from build123d import *

# Parameters (mm, degrees)
SKETCH1_R           = 3.06
BOSS_EXTRUDE1_DEPTH = 2
BOSS_EXTRUDE3_DEPTH = 5
SKETCH6_W           = 56
SKETCH6_H           = 2
BOSS_EXTRUDE4_DEPTH = 2
FILLET2_R           = 30
FILLET3_R           = 4


with BuildPart() as part:
    # Sketch1 → Boss-Extrude1 (new body)
    with BuildSketch(Plane(origin=(0, 0, 0), x_dir=(1, 0, 0), z_dir=(0, 1, 0))):
        with BuildLine():
            Line((-5, 0), (-5, 5))
            Line((-5, 5), (71, 5))
            Line((71, 5), (71, -3))
            ThreePointArc((71, -3), (66, -8), (61, -3))
            Line((61, -3), (61, 3.06))
            Line((61, 3.06), (5, 3.06))
            Line((5, 3.06), (5, 0))
            ThreePointArc((5, 0), (0, -5), (-5, 0))
        make_face()
        with Locations(Location((0, 0, 0), (0, 0, 270))):
            Circle(SKETCH1_R, mode=Mode.SUBTRACT)
        with Locations(Location((66, -3, 0), (0, 0, 270))):
            Circle(SKETCH1_R, mode=Mode.SUBTRACT)
    extrude(amount=BOSS_EXTRUDE1_DEPTH)

    # Sketch4 → Boss-Extrude3 (add)
    with BuildSketch(Plane(origin=(0, 0, 0), x_dir=(-1, 0, 0), z_dir=(0, -1, 0))):
        Polygon((5, 5), (-71, 5), (-89.933264969, -12.968832246), (-66.5, 3.06), (5, 3.06), align=None)
    extrude(amount=BOSS_EXTRUDE3_DEPTH)

    # Sketch6 → Boss-Extrude4 (add)
    with BuildSketch(Plane(origin=(0, 2, 0), x_dir=(1, 0, 0), z_dir=(0, 1, 0))):
        with Locations((33, 2.06)):
            Rectangle(SKETCH6_W, SKETCH6_H)
    extrude(amount=-BOSS_EXTRUDE4_DEPTH)

    # Fillet2
    # the kernel refuses this fillet: 30 mm, written as the material it takes off along each edge
    with BuildSketch(Plane(origin=(71, 29.924182181, -5), x_dir=(0.7253392750671382, 0, 0.6883915572151349), z_dir=(0, -1, 0))) as fillet2_piece_1:
        with BuildLine():
            CenterArc((FILLET2_R * 0.398989095747, FILLET2_R), FILLET2_R, 226.497078838, 43.502921162)
            Line((-FILLET2_R * 0.289402461469, FILLET2_R * 0.274660724933), (0, 0))
            Line((0, 0), (FILLET2_R * 0.398989095747, 0))
        make_face()
    extrude(amount=64.848364362, mode=Mode.SUBTRACT)

    # Fillet3
    # the kernel refuses this fillet: 4 mm, written as the material it takes off along each edge
    with BuildSketch(Plane(origin=(-5, 12, -5), x_dir=(0, 0, 1), z_dir=(0, -1, 0))) as fillet3_piece_1:
        with BuildLine():
            CenterArc((FILLET3_R, -FILLET3_R), FILLET3_R, 90, 90)
            Line((0, -FILLET3_R), (0, 0))
            Line((0, 0), (FILLET3_R, 0))
        make_face()
    extrude(amount=27, mode=Mode.SUBTRACT)


solid = part.part
Verification items for the finished model (mm, model axes). A direction names the side the tool comes from. Round coordinates to 2 decimals unless told otherwise and drop trailing zeros. Loops run counter-clockwise (first coordinate to the right, second up) from the corner with the lowest first, then second, coordinate; pieces in that order, holes last. Notation, with made-up numbers: M -31,-9.75 L -7,-9.75 A20 cw -7,9.25 Z; hole C -36,-35.75 d1. An arc over 180 degrees is marked long. Write each question's results on one line, items separated by ' | '.
1) Scan lines: L1, parallel to Z at x = 15, y = -2.75; L2, parallel to Y at x = 63, z = -3; L3, parallel to X at y = 1, z = 3.25. Record each from-to range of solid material in increasing order. Write a range as from..to.
Checks:
L1: z = -5..-3.06 | L2: y = 0..2 | L3: x = -3.8..3.8, 61.01..62.95, 69.05..70.99
2) Access from +Z, -Z, +X, -X, +Y, -Y to the whole of each face (thin tool, end or side, straight path). Record for faces 1 (the flat face through (36, 0, -2)), 2 (the cylindrical face through (-2.99, 0.99, -0.66)), 3 (the flat face through (78, 0, 3)), 4 (the flat face through (33, 1, -1.06)).
Checks:
face 1: +Z, -X, -Y | face 2: +Y, -Y | face 3: +Z, -Z, +X, +Y | face 4: +Z, +Y, -Y
3) Section check A-A on z = 7. Record the boundary of the cut face in (x, y), then the cut area to 3 significant figures.
Checks:
outline: M 63,0 L 69,0 L 69,2 L 63,2 Z; M 81.21,-5 L 83.64,-5 L 83.64,0 L 81.21,0 Z | area: 24.2 mm2
4) Section check D-D on x = 80.5. Record the boundary of the cut face in (y, z).
Checks:
outline: M -5,4.02 L 0,4.02 L 0,6.52 L -5,6.52 Z
5) Mould release check, pull along Z, two halves, no side actions. Record for faces 5 (the cylindrical face through (63.01, 0.99, 2.34)), 6 (the flat face through (71, 1, 0)), 7 (the flat face through (78.381, -2.465, 5.067)): released by +Z, released by -Z, zero draft, split by the parting line, or undercut.
Checks:
face 5: undercut | face 6: zero draft | face 7: released by +Z
6) Section check C-C on y = -1. Record the boundary of the cut face in (x, z).
Checks:
outline: M -4.43,-3.06 A4 ccw -1,-5 L 59.03,-5 A30 ccw 79.68,3.24 L 89.93,12.97 L 66.5,-3.06 Z
7) Section check B-B on x = 26. Record the boundary of the cut face in (y, z), then the cut area to 3 significant figures.
Checks:
outline: M -5,-5 L 2,-5 L 2,-1.06 L 0,-1.06 L 0,-3.06 L -5,-3.06 Z | area: 17.6 mm2
8) Gauge pin test, flat ends, axial feed: P1, Ø1.5, axis at x = 34.5, y = -2, coming from the +Z side; P2, Ø4, axis at y = -3.5, z = 0.5, coming from the +X side; P3, Ø4.5, axis at x = 83.5, z = 1.5, coming from the +Y side; P4, Ø1.6, axis at y = 1.5, z = 0.5, coming from the -X side. Record the tip position at first contact, or that the pin passes through.
Checks:
P1: stops at z = -3.06 | P2: stops at x = 78.87 | P3: passes through | P4: stops at x = -5
